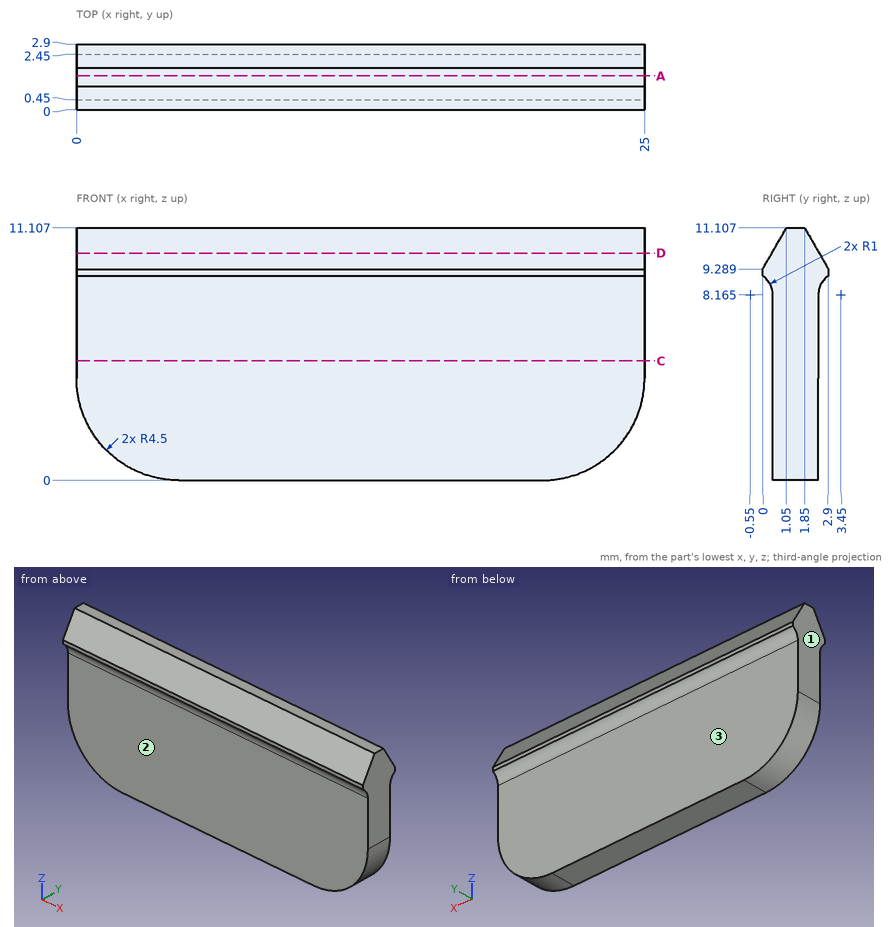
Print and shaded views of the part. All mm, measured from the part's lowest x, y and z. A direction names the side the tool comes from. Give positions to 0.01 mm unless a question says otherwise; leave off trailing zeros. Write each loop counter-clockwise with the first axis right and the second up, starting at its lowest first coordinate (ties: lowest second). Pieces come first, ordered by that corner, then holes. Notation, with made-up numbers: (-37, 78.5) -> (21, 78.5) arc R13 ccw to (21, 94.5) -> close; hole circle Ø6 at (36.25, -35.75). An arc over 180 degrees is marked (long way). Use CSV: the item, a comma, the result in double quotes. Start each with the question number.
1) Pin check, flat tips, straight feed: P1, Ø4, axis at x = 9.5, z = 2.5, coming from the +Y side; P2, Ø4, axis at x = 18.5, z = 4.5, coming from the -Y side. Stop position of each tip, or through.
2) Tool access for the marked faces 1, 2 and 3: list every direction of +Z, -Z, +X, -X, +Y, -Y with a clear straight run to the whole face (end or side of a thin tool).
3) Cut at A-A on y = 1.5. List the corners of the cut face in (x, z).
4) Cut at C-C on z = 5.25. List the corners of the cut face in (x, y).
5) Drill centre lines: L1, parallel to Y at x = 17.5, z = 3.5; L2, parallel to X at y = 2.2, z = 2.75 (1 decimal); L3, parallel to Z at x = 7, y = 0.95 (1 decimal). Where is each one in solid material? Low to high.
6) Cut at D-D on z = 10. List the corners of the cut face in (x, y).
Final values:
1,P1,"stops at y = 2.45"
1,P2,"stops at y = 0.45"
2,face 1,"+Z, -Z, -X, +Y, -Y"
2,face 2,"-Z, +X, -X, -Y"
2,face 3,"-Z, +X, -X, +Y"
3,outline,"(0, 4.5) arc R4.5 ccw to (4.5, 0) -> (20.5, 0) arc R4.5 ccw to (25, 4.5) -> (25, 11.11) -> (0, 11.11) -> close"
4,outline,"(0, 0.45) -> (25, 0.45) -> (25, 2.45) -> (0, 2.45) -> close"
5,L1,"y = 0.45 to 2.45"
5,L2,"x = 0.4 to 24.6"
5,L3,"z = 0 to 10.9"
6,outline,"(0, 0.41) -> (25, 0.41) -> (25, 2.49) -> (0, 2.49) -> close"
